from build123d import *

# Parameters (mm, degrees)
SKETCH1_R           = 2.465
BOSS_EXTRUDE1_DEPTH = 2.9
SKETCH2_R           = 1.45
BOSS_EXTRUDE2_DEPTH = 10
CUT_EXTRUDE1_DEPTH  = 1.9
CHAMFER1_SIZE       = 0.25


with BuildPart() as part:
    # Sketch1 → Boss-Extrude1 (new body)
    with BuildSketch(Plane(origin=(0, 0, 0), x_dir=(1, 0, 0), z_dir=(0, 1, 0))):
        Circle(SKETCH1_R)
    extrude(amount=BOSS_EXTRUDE1_DEPTH)

    # Sketch2 → Boss-Extrude2 (add)
    with BuildSketch(Plane(origin=(0, 2.9, 0), x_dir=(1, 0, 0), z_dir=(0, 1, 0))):
        Circle(SKETCH2_R)
    extrude(amount=BOSS_EXTRUDE2_DEPTH)

    # Sketch3 → Cut-Extrude1 (cut)
    with BuildSketch(Plane.XZ):
        Polygon((0.733234842, -1.27), (1.466469684, 0), (0.733234842, 1.27), (-0.733234842, 1.27), (-1.466469684, 0), (-0.733234842, -1.27), align=None)
    extrude(amount=-CUT_EXTRUDE1_DEPTH, mode=Mode.SUBTRACT)

    # Chamfer1
    chamfer1_edges = [part.edges().sort_by_distance(p)[0] for p in [
        (-1.45, 12.9, 0),
    ]]
    chamfer(chamfer1_edges, length=CHAMFER1_SIZE)


solid = part.part
Here's how the part is built. I have some questions about the finished solid (model axes, mm). A direction names the side the tool comes from. Coordinates: 2 decimals unless noted, no trailing zeros. Write each loop counter-clockwise with the first axis right and the second up, starting at its lowest first coordinate (ties: lowest second). Pieces come first, ordered by that corner, then holes.
Item 1: I want a section at C-C on x = 1.7. Write out the boundary of the cut face in (y, z) (3 decimals).
Item 2: If I drill on line 1 (Y direction, x = -0.15, z = 1.6); line 2 (Y direction, x = -0.55, z = 0.5); line 3 (Z direction, x = -0.7, y = 7), over which ranges is the centre line in solid material (lowest first)?
Item 3: I want a section at B-B on y = 3.5. Write out the boundary of the cut face in (x, z).
Item 4: If we mould it in two halves opening along X, with no side actions, what happens to faces 1 (the cylindrical face through (-1.956, 1.43, 1.5)), 2 (the flat face through (0, 1, 1.27)), 3 (the flat face through (1.095, 0.937, -0.644)), 4 (the flat face through (0, 2.9, 2))? For each: +X half, -X half, draft (parallel to the pull), parting line (faces both ways), or undercut.
Item 5: On a 3-axis mill with a long thin cutter (end or side, diameter ignored), from which of +Z, -Z, +X, -X, +Y, -Y can I reach the whole of each face in a straight line? I mean faces 5 (the cylindrical face through (-1.45, 7.71, -0.06)), 6 (the flat face through (0, 12.9, 0)), 7 (the flat face through (-1.105, 0.937, -0.626)). Say none if no direction works.
Item 6: Will these pins go through, and if not, where does the flat tip stop? pin 1 (1 mm diameter, centred on x = -0.5, y = 5.5, fed in from -Z); pin 2 (1 mm diameter, centred on x = 1.5, z = 0.5, fed in from -Y); pin 3 (0.8 mm diameter, centred on x = -0.5, z = -0.5, fed in from -Y).
Item 7: I want a section at A-A on x = 0. Write out the boundary of the cut face in (y, z) (3 decimals), and give its area (3 significant figures).
Findings below:
1. outline: (0, -1.785) - (2.9, -1.785) - (2.9, 1.785) - (0, 1.785) - close
2. line 1: y = 0 to 2.9
2. line 2: y = 1.9 to 12.9
2. line 3: z = -1.27 to 1.27
3. outline: circle Ø2.9 at (0, 0)
4. face 1: parting line
4. face 2: undercut
4. face 3: undercut
4. face 4: draft
5. face 5: +Y
5. face 6: +Z, -Z, +X, -X, +Y
5. face 7: -Y
6. pin 1: stops at z = -1.45
6. pin 2: stops at y = 0
6. pin 3: stops at y = 1.9
7. outline: (0, -2.465) - (2.9, -2.465) - (2.9, -1.45) - (12.65, -1.45) - (12.9, -1.2) - (12.9, 1.2) - (12.65, 1.45) - (2.9, 1.45) - (2.9, 2.465) - (0, 2.465) - (0, 1.27) - (1.9, 1.27) - (1.9, -1.27) - (0, -1.27) - close
7. area: 38.4 mm2
